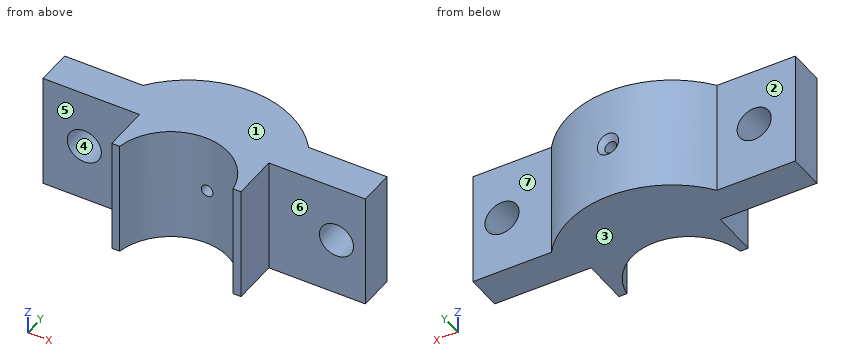
from build123d import *

# Parameters (mm, degrees)
BOSS_EXTRUDE1_DEPTH                                 = 64
F_1_0MM_DOWEL_HOLE1_D                               = 19
F_1_0MM_DOWEL_HOLE1_DEPTH                           = 130
F_1_0MM_DOWEL_HOLE1_TIP                             = 5.708175881
CSK_FOR_M6_COUNTERSUNK_FLAT_HEAD_SCREW1_D           = 6.6
CSK_FOR_M6_COUNTERSUNK_FLAT_HEAD_SCREW1_DEPTH       = 130
CSK_FOR_M6_COUNTERSUNK_FLAT_HEAD_SCREW1_CSINK_D     = 12.6
CSK_FOR_M6_COUNTERSUNK_FLAT_HEAD_SCREW1_CSINK_ANGLE = 90
CSK_FOR_M6_COUNTERSUNK_FLAT_HEAD_SCREW1_TIP         = 1.982840043


with BuildPart() as part:
    # Sketch1 → Boss-Extrude1 (new body)
    with BuildSketch(Plane.XY):
        with BuildLine():
            Line((0, 0), (0, 20))
            Line((0, 20), (43.660658251, 20))
            ThreePointArc((43.660658251, 20), (89.797593381, 42.851981325), (135.934528511, 20))
            Line((135.934528511, 20), (179.595186762, 20))
            Line((179.595186762, 20), (179.595186762, 0))
            Line((179.595186762, 0), (125.797593381, 0))
            Line((125.797593381, 0), (125.797593381, -25.778358914))
            Line((125.797593381, -25.778358914), (121.37101897, -25.778358914))
            ThreePointArc((121.37101897, -25.778358914), (89.797593381, 1.014070006), (58.224167792, -25.778358914))
            Line((58.224167792, -25.778358914), (53.797593381, -25.778358914))
            Line((53.797593381, -25.778358914), (53.797593381, 0))
            Line((53.797593381, 0), (0, 0))
        make_face()
    extrude(amount=BOSS_EXTRUDE1_DEPTH)

    # Ø1.0mm Dowel Hole1
    with Locations(Plane(origin=(0, 20, 0), x_dir=(1, 0, 0), z_dir=(0, 1, 0))):
        with Locations((22.988007273, -32), (163.454699395, -32.277602158)):
            Hole(F_1_0MM_DOWEL_HOLE1_D / 2, depth=F_1_0MM_DOWEL_HOLE1_DEPTH)
            with Locations((0, 0, -(F_1_0MM_DOWEL_HOLE1_DEPTH + F_1_0MM_DOWEL_HOLE1_TIP / 2))):  # 118° drill point
                Cone(0, F_1_0MM_DOWEL_HOLE1_D / 2, F_1_0MM_DOWEL_HOLE1_TIP, mode=Mode.SUBTRACT)

    # CSK for M6 Countersunk Flat Head Screw1
    with Locations(Plane(origin=(0, 42.851981325, 0), x_dir=(1, 0, 0), z_dir=(0, 1, 0))):
        with Locations((90.934528511, -32)):
            CounterSinkHole(CSK_FOR_M6_COUNTERSUNK_FLAT_HEAD_SCREW1_D / 2, CSK_FOR_M6_COUNTERSUNK_FLAT_HEAD_SCREW1_CSINK_D / 2, depth=CSK_FOR_M6_COUNTERSUNK_FLAT_HEAD_SCREW1_DEPTH, counter_sink_angle=CSK_FOR_M6_COUNTERSUNK_FLAT_HEAD_SCREW1_CSINK_ANGLE)
            with Locations((0, 0, -(CSK_FOR_M6_COUNTERSUNK_FLAT_HEAD_SCREW1_DEPTH + CSK_FOR_M6_COUNTERSUNK_FLAT_HEAD_SCREW1_TIP / 2))):  # 118° drill point
                Cone(0, CSK_FOR_M6_COUNTERSUNK_FLAT_HEAD_SCREW1_D / 2, CSK_FOR_M6_COUNTERSUNK_FLAT_HEAD_SCREW1_TIP, mode=Mode.SUBTRACT)


solid = part.part
Part model, mm, in its own coordinate system. Face numbers are marked on the shaded views. A direction names the side the tool comes from. Coordinates: 2 decimals unless noted, no trailing zeros. Loops run counter-clockwise (first coordinate to the right, second up) from the corner with the lowest first, then second, coordinate; pieces in that order, holes last. Notation, with made-up numbers: M 48,30.25 L 89,30.25 A20 cw 89,36.25 Z; hole C 43,64.25 d7. An arc over 180 degrees is marked long. Use a Markdown table: item, result. Add a question column.
Q1. Cut at C-C (z = 5). Write the cut outline in (x, y), and give its area (3 significant figures).
Q2. Pin check, flat tips, straight feed: P1, Ø10, axis at x = 22.5, z = 46, coming from the -Y side; P2, Ø13, axis at x = 16, z = 37, coming from the +Y side; P3, Ø20.5, axis at y = -11, z = 28.5, coming from the +X side; P4, Ø15, axis at x = 22.99, z = 32, coming from the +Y side. Stop position of each tip, or through.
Q3. Mould opens along Z. For the marked faces 1, 2, 3 and 4 say: +Z half, -Z half, draft (parallel to the pull), parting line (faces both ways), or undercut.
Q4. Cut at B-B (x = 163). Write the cut outline in (y, z), and give its area (3 significant figures).
Q5. Cut at D-D (y = 37.5). Write the cut outline in (x, z).
Q6. Cut at A-A (y = -4.5). Write the cut outline in (x, z), and give its area (3 significant figures).
Q7. Probe L1, parallel to X at y = 18.5, z = 32; L2, parallel to X at y = 12, z = 27.5; L3, parallel to Y at x = 151, z = 7. List the from-to ranges inside material, lowest first.
Q8. Which spindle directions (+Z, -Z, +X, -X, +Y, -Y) get a long thin tool onto all of the face, cutting with end or side? Do the marked faces 5, 6 and 7. Say none if no direction does.
Worked out:
| question | item | result |
|---|---|---|
| 1 | outline | M 0,0 L 53.8,0 L 53.8,-25.78 L 58.22,-25.78 A32 cw 121.37,-25.78 L 125.8,-25.78 L 125.8,0 L 179.6,0 L 179.6,20 L 135.93,20 A58 ccw 43.66,20 L 0,20 Z |
| 1 | area | 5,640 mm2 |
| 2 | P1 | stops at y = 0 |
| 2 | P2 | stops at y = 20 |
| 2 | P3 | stops at x = 125.8 |
| 2 | P4 | passes through |
| 3 | face 1 | +Z half |
| 3 | face 2 | draft |
| 3 | face 3 | -Z half |
| 3 | face 4 | undercut |
| 4 | outline | M 0,0 L 20,0 L 20,22.79 L 0,22.79 Z; M 0,41.77 L 20,41.77 L 20,64 L 0,64 Z |
| 4 | area | 900 mm2 |
| 5 | outline | M 65.46,0 L 114.13,0 L 114.13,64 L 65.46,64 Z; hole C 90.93,32 d6.6 |
| 6 | outline | M 53.8,0 L 71.84,0 L 71.84,64 L 53.8,64 Z; M 107.76,0 L 125.8,0 L 125.8,64 L 107.76,64 Z |
| 6 | area | 2,310 mm2 |
| 7 | L1 | x = 0 to 13.49, 32.49 to 87.63, 94.23 to 153.96, 172.95 to 179.6 |
| 7 | L2 | x = 0 to 14.62, 31.35 to 155.24, 171.67 to 179.6 |
| 7 | L3 | y = 0 to 20 |
| 8 | face 5 | +Z, -Z, -X, -Y |
| 8 | face 6 | +Z, -Z, +X, -Y |
| 8 | face 7 | +Z, -Z, +X, +Y |
